```python
from build123d import *

# Parameters (mm, degrees)
BOSS_EXTRUDE1_DEPTH = 4
CUT_EXTRUDE1_DEPTH  = 5
CUT_EXTRUDE2_DEPTH  = 10
SKETCH4_W           = 8
SKETCH4_H           = 4
BOSS_EXTRUDE2_DEPTH = 4


with BuildPart() as part:
    # Sketch1 → Boss-Extrude1 (new body)
    with BuildSketch(Plane.XY):
        Polygon((20.5, -41), (20.5, -26), (-20.5, -26), (-20.5, -41), (-55, -41), (-55, 41), (-15, 41), (-15, 45), (15, 45), (15, 41), (55, 41), (55, -41), align=None)
    extrude(amount=BOSS_EXTRUDE1_DEPTH)

    # Sketch2 → Cut-Extrude1 (cut)
    with BuildSketch(Plane(origin=(0, 0, 0), x_dir=(-1, 0, 0), z_dir=(0, 0, -1))):
        Polygon((-41, -36), (-41, -41), (-45, -41), (-45, -36), (-46.5, -36), (-46.5, -32.8), (-45, -32.8), (-45, -20), (-41, -20), (-41, -32.8), (-39.5, -32.8), (-39.5, -36), align=None)
        Polygon((45, -41), (45, -36), (46.5, -36), (46.5, -32.8), (45, -32.8), (45, -20), (41, -20), (41, -32.8), (39.5, -32.8), (39.5, -36), (41, -36), (41, -41), align=None)
        Polygon((41, 36), (41, 41), (45, 41), (45, 36), (46.5, 36), (46.5, 32.8), (45, 32.8), (45, 20), (41, 20), (41, 32.8), (39.5, 32.8), (39.5, 36), align=None)
        Polygon((-45, 41), (-45, 36), (-46.5, 36), (-46.5, 32.8), (-45, 32.8), (-45, 20), (-41, 20), (-41, 32.8), (-39.5, 32.8), (-39.5, 36), (-41, 36), (-41, 41), align=None)
    extrude(amount=-CUT_EXTRUDE1_DEPTH, mode=Mode.SUBTRACT)

    # Sketch3 → Cut-Extrude2 (cut)
    with BuildSketch(Plane(origin=(0, 0, 0), x_dir=(-1, 0, 0), z_dir=(0, 0, -1))):
        with BuildLine():
            ThreePointArc((-27.96981837, -8.015850853), (-31.5, -4.536419435), (-35.03018163, -8.015850853))
            ThreePointArc((-35.03018163, -8.015850853), (-37.984301772, -11), (-35.03018163, -13.984149147))
            ThreePointArc((-35.03018163, -13.984149147), (-31.5, -17.463580565), (-27.96981837, -13.984149147))
            ThreePointArc((-27.96981837, -13.984149147), (-25.015698228, -11), (-27.96981837, -8.015850853))
        make_face()
        with BuildLine():
            ThreePointArc((35.03018163, -8.015850853), (37.984301772, -11), (35.03018163, -13.984149147))
            ThreePointArc((35.03018163, -13.984149147), (31.5, -17.463580565), (27.96981837, -13.984149147))
            ThreePointArc((27.96981837, -13.984149147), (25.015698228, -11), (27.96981837, -8.015850853))
            ThreePointArc((27.96981837, -8.015850853), (31.5, -4.536419435), (35.03018163, -8.015850853))
        make_face()
    extrude(amount=-CUT_EXTRUDE2_DEPTH, mode=Mode.SUBTRACT)

    # Sketch4 → Boss-Extrude2 (add)
    with BuildSketch(Plane(origin=(0, 0, 0), x_dir=(-1, 0, 0), z_dir=(0, 0, -1))):
        with Locations((-31, -43)):
            Rectangle(SKETCH4_W, SKETCH4_H)
        with Locations((31, -43)):
            Rectangle(SKETCH4_W, SKETCH4_H)
    extrude(amount=-BOSS_EXTRUDE2_DEPTH)


solid = part.part
```
Verification items for the finished model (mm, model axes). A direction names the side the tool comes from. Round coordinates to 2 decimals unless told otherwise and drop trailing zeros. Write each loop counter-clockwise with the first axis right and the second up, starting at its lowest first coordinate (ties: lowest second). Pieces come first, ordered by that corner, then holes. Notation, with made-up numbers: (50, 82.5) -> (105, 82.5) arc R33 cw to (105, 110.5) -> close; hole circle Ø5 at (-34.5, 22). An arc over 180 degrees is marked (long way). Write each question's results on one line, items separated by ' | '. Start each with the question number.
1. Set-up check for faces 4 (the flat face through (-43, 20, 2)), 5 (the flat face through (-45, -39, 2)), 6 (the cylindrical face through (31.577, -17.463, 1.972)): record each of +Z, -Z, +X, -X, +Y, -Y from which the full face is reachable in a straight line by a thin tool's end or side.
2. Cross-section at D-D (y = 26.5). Enter the section's corners in (x, z), then the cut area to 3 significant figures.
3. Depth check by flat-ended pin: P1, Ø1, axis at x = -2.5, z = 0.5, coming from the -Y side; P2, Ø0.8, axis at x = 40, z = 3, coming from the +Y side; P3, Ø1.5, axis at x = -22, z = 1.5, coming from the -Y side. Enter the tip coordinate at first touch or a pass-through.
4. Cross-section at B-B (y = -11). Enter the section's corners in (x, z), then the cut area to 3 significant figures.
5. Draft check along Y on faces 1 (the flat face through (-45, 26, 2)), 2 (the flat face through (39.5, 34, 2)), 3 (the flat face through (50, -41, 2)). Enter one of: +Y half, -Y half, draft (parallel to the pull), parting line (faces both ways), or undercut.
6. Cross-section at C-C (z = 2.05). Count the separate pieces of the cut face and the enclosed holes in it, then the cut area to 3 significant figures.
7. Cross-section at A-A (x = 31.5). Enter the section's corners in (y, z).
8. Material ranges on probe 1 along X at (y, z) = (-11, 3.5); probe 2 along X at (y, z) = (-33.5, 1.5); probe 3 along X at (y, z) = (31.5, 0.7), recorded low to high. Write a range as from..to.
Solutions:
1) face 4: +Z, -Z, +Y | face 5: +Z, -Z, -Y | face 6: +Z, -Z
2) outline: (-55, 0) -> (-45, 0) -> (-45, 4) -> (-55, 4) -> close; (-41, 0) -> (41, 0) -> (41, 4) -> (-41, 4) -> close; (45, 0) -> (55, 0) -> (55, 4) -> (45, 4) -> close | area: 408 mm2
3) P1: stops at y = -26 | P2: stops at y = 41 | P3: stops at y = -41
4) outline: (-55, 0) -> (-37.98, 0) -> (-37.98, 4) -> (-55, 4) -> close; (-25.02, 0) -> (25.02, 0) -> (25.02, 4) -> (-25.02, 4) -> close; (37.98, 0) -> (55, 0) -> (55, 4) -> (37.98, 4) -> close | area: 336 mm2
5) face 1: draft | face 2: undercut | face 3: -Y half
6) separate pieces: 1 | enclosed holes: 2 | area: 8,000 mm2
7) outline: (-45, 0) -> (-17.46, 0) -> (-17.46, 4) -> (-45, 4) -> close; (-4.54, 0) -> (41, 0) -> (41, 4) -> (-4.54, 4) -> close
8) probe 1: x = -55..-37.98, -25.02..25.02, 37.98..55 | probe 2: x = -55..-46.5, -39.5..-20.5, 20.5..39.5, 46.5..55 | probe 3: x = -55..-45, -41..41, 45..55
